Design review of the part built by this model. Coordinates are the model's own, in mm. A direction names the side the tool comes from. Coordinates: 2 decimals unless noted, no trailing zeros. Loops run counter-clockwise (first coordinate to the right, second up) from the corner with the lowest first, then second, coordinate; pieces in that order, holes last. Notation, with made-up numbers: (40, 56) -> (61, 56) arc R35 ccw to (61, 92) -> close; hole circle Ø1 at (80.25, 45). An arc over 180 degrees is marked (long way). Answer in a Markdown table with one row per item.
Autodesk Inventor part; units mm, degrees
ref_plane "YZ Plane" through (0, 0, 0) normal (1, 0, 0) x (0, 1, 0)
ref_plane "XZ Plane" through (0, 0, 0) normal (0, 1, 0) x (-1, 0, 0)
ref_plane "XY Plane" through (0, 0, 0) normal (0, 0, 1) x (1, 0, 0)
sketch "Sketch1" plane through (0, 0, 0) normal (0, 1, 0) x (-1, 0, 0)
  line L0 (0, 0) -> (47.625, 0)
  line L1 (47.625, 0) -> (47.625, -50.165)
  line L2 (47.625, -50.165) -> (0, -50.165)
  line L3 (0, -50.165) -> (0, 0)
  dimension "d0" = 47.625
  dimension "d1" = 50.165
extrude "Extrusion1" add sketch "Sketch1" along normal blind 2.54
sketch "Sketch2" plane through (0, 2.54, 0) normal (0, 1, 0) x (1, 0, 0)
  line L0 (-47.625, 0) -> (0, 0)
  line L1 (0, 0) -> (-2.54, 0)
  line L2 (-2.54, 0) -> (-2.54, 2.54)
  line L3 (-2.54, 2.54) -> (0, 2.54)
  line L4 (0, 2.54) -> (0, 0)
  line L5 (0, 0) -> (0, 50.165)
  line L6 (0, 50.165) -> (-2.54, 50.165)
  line L7 (-2.54, 50.165) -> (-2.54, 47.625)
  line L8 (-2.54, 47.625) -> (0, 47.625)
  line L9 (0, 47.625) -> (0, 50.165)
  line L10 (-47.625, 50.165) -> (-47.625, 0)
  line L11 (-47.625, 50.165) -> (-45.085, 50.165)
  line L12 (-45.085, 50.165) -> (-45.085, 47.625)
  line L13 (-45.085, 47.625) -> (-47.625, 47.625)
  line L14 (-47.625, 47.625) -> (-47.625, 50.165)
  line L15 (-47.625, 0) -> (-45.085, 0)
  line L16 (-45.085, 0) -> (-45.085, 2.54)
  line L17 (-45.085, 2.54) -> (-47.625, 2.54)
  line L18 (-47.625, 2.54) -> (-47.625, 0)
  dimension "d4" = 2.54
  dimension "d5" = 2.54
  dimension "d6" = 2.54
  dimension "d7" = 2.54
hole "Hole1" at (-45.085, 2.54, -47.625) at (-2.54, 2.54, -47.625) at (-2.54, 2.54, -2.54) at (-45.085, 2.54, -2.54) direction (0, -1, 0) diameter 3.2766 depth 7.2771 counterbore diameter 5.5626 counterbore depth 1.5875
fillet "Fillet1" radius 3.175 4 edges at (-23.8125, 2.54, 0) (0, 2.54, -25.0825) (-23.8125, 2.54, -50.165) (-47.625, 2.54, -25.0825)
properties part number "Lid-SensorHousing"
(1) To check wall thickness, follow probe 1 along X at (y, z) = (0.7, -2.54); probe 2 along X at (y, z) = (0.1, -46.5); probe 3 along Z at (x, y) = (-2.54, 0.35). State the ranges of each line that lie inside material, in increasing order.
Evaluation:
| item | result |
|---|---|
| probe 1 | x = -47.39 to -46.72, -43.45 to -4.18, -0.9 to -0.23 |
| probe 2 | x = -47.6 to -46.28, -43.89 to -3.73, -1.35 to -0.02 |
| probe 3 | z = -50.07 to -49.26, -45.99 to -4.18, -0.9 to -0.09 |
(2) Take a section at C-C on y = 0.4. Give the boundary of the cut face in (x, z) (3 decimals).
Evaluation:
| item | result |
|---|---|
| outline | (-47.516, -50.056) -> (-0.109, -50.056) -> (-0.109, -0.109) -> (-47.516, -0.109) -> close; hole circle Ø3.277 at (-45.085, -47.625); hole circle Ø3.277 at (-45.085, -2.54); hole circle Ø3.277 at (-2.54, -47.625); hole circle Ø3.277 at (-2.54, -2.54) |
(3) Tool access review of faces 5 (the cylindrical face through (-4.46, 1.74, -45.61)), 6 (the cylindrical face through (-46.466, 0.47, -46.744)): name each direction out of +Z, -Z, +X, -X, +Y, -Y from which nothing blocks a thin tool from reaching the whole face with its end or side.
Evaluation:
| item | result |
|---|---|
| face 5 | +Y |
| face 6 | +Y, -Y |
(4) Take a section at D-D on z = -24.5. Give the boundary of the cut face in (x, y) (3 decimals).
Evaluation:
| item | result |
|---|---|
| outline | (-47.625, 0) -> (0, 0) arc R3.175 ccw to (-3.111, 2.54) -> (-44.514, 2.54) arc R3.175 ccw to start |
(5) Draft analysis for pull direction Z (two halves, no side actions). For faces 1 (the cylindrical face through (-23.479, 1.843, -1.126)), 2 (the cylindrical face through (-3.03, 0.47, -46.06)), 3 (the flat face through (-24, 2.54, -25)), 4 (the flat face through (-4, 0.952, -46)), state which applies: pulls with the +Z half, pulls with the -Z half, needs draft (parallel to the pull), parting line crosses it, or undercut.
Evaluation:
| item | result |
|---|---|
| face 1 | pulls with the +Z half |
| face 2 | undercut |
| face 3 | needs draft |
| face 4 | undercut |
(6) Take a section at A-A on z = -2.54. Count the separate pieces of the cut face and the enclosed holes in it, and give its area (3 significant figures).
Evaluation:
| item | result |
|---|---|
| separate pieces | 3 |
| enclosed holes | 0 |
| area | 95.6 mm² |
(7) For pin 1 (1.5 mm diameter, centred on x = -3.5, z = -2, fed in from +Y); pin 2 (5.5 mm diameter, centred on x = -45.5, z = -1.5, fed in from +Y); pin 3 (1.5 mm diameter, centred on x = -19, y = 1.5, fed in from -Z), all flat-tipped, find the tip position at first contact; note any pin that passes through.
Evaluation:
| item | result |
|---|---|
| pin 1 | stops at y = 0.95 |
| pin 2 | stops at y = 1.69 |
| pin 3 | stops at z = -49.91 |
